Here's how the part is built. I have some questions about the finished solid (model axes, mm). A direction names the side the tool comes from. Coordinates: 2 decimals unless noted, no trailing zeros. Order: outer loops, then holes, each group sorted by start corner. A loop starts at its lowest first (then second) coordinate and runs counter-clockwise, first axis right, second up.
```python
from build123d import *

# Parameters (mm, degrees)
F1_DEPTH = 19.05
F2_W     = 44.4994677836
F2_H     = 19.1223323345
F3_DEPTH = 63.5
F5_DEPTH = 19.05
F6_DEPTH = 19.05


with BuildPart() as f1:
    # F0 (on Right) → F1 (new body)
    with BuildSketch(Plane.YZ):
        Polygon((-30.6730988776, 12.7), (-30.6730988776, 0), (32.876368906, 0), (32.876368906, 44.45), (13.826368906, 44.45), align=None)
    extrude(amount=F1_DEPTH)

    # F2 (on face) → F3 (join)
    with BuildSketch(Plane.YZ.offset(19.05)):
        with Locations((10.6266350142, 9.5611661673)):
            Rectangle(F2_W, F2_H)
    extrude(amount=F3_DEPTH)

    # F4 (on face) → F5 (join)
    with BuildSketch(Plane.YZ.offset(82.55)):
        Polygon((-11.6230988776, 19.1223323345), (32.876368906, 19.1223323345), (32.876368906, 44.45), (13.826368906, 44.45), (-30.623631094, 12.7), (-30.623631094, 0), (-11.6230988776, 0), align=None)
    extrude(amount=F5_DEPTH)

    # F6 (add, through all): a face of the model
    f6_faces = [f1.faces().sort_by_distance(p)[0] for p in [
        (82.55, 10.6266350142, 9.5611661673),
    ]]
    extrude(f6_faces, amount=F6_DEPTH)


solid = f1.part
```
Q1. If we section it at D-D on z = 10.5: Write out the boundary of the cut face in (x, y).
Q2. We'd pull the mould along X, two halves only. Please class faces 1 (the flat face through (101.6, 8, 18)), 2 (the flat face through (50, 10, 19.122)), 3 (the flat face through (50, 8, 0)): pulls with the +X half, pulls with the -X half, needs draft (parallel to the pull), parting line crosses it, or undercut.
Q3. For faces 4 (the flat face through (92, 23, 44.45)), 5 (the flat face through (50, -11.623, 9)), 6 (the flat face through (19.05, 1, 23)), which set-ups out of +Z, -Z, +X, -X, +Y, -Y let a thin tool reach every point of the face, with its end or its side?
Q4. If we section it at C-C on x = 94: Write out the boundary of the cut face in (y, z), then the cut area to 3 significant figures.
Q5. I need wall thicknesses on L1, parallel to X at y = 5, z = 27; L2, parallel to Y at x = 64.5, z = 3; L3, parallel to Z at x = 73, y = 11.5. Which ranges of each line are inside material? Lowest first, please.
Q6. If we section it at A-A on z = 40.5: Write out the boundary of the cut face in (x, y).
Q7. If we section it at B-B on y = 15.5: Write out the boundary of the cut face in (x, z).
Q8. Will these pins go through, and if not, where does the flat tip stop? pin 1 (15.5 mm diameter, centred on x = 52.5, z = 10, fed in from -Y); pin 2 (12 mm diameter, centred on x = 84, z = 14.5, fed in from -Y).
Reply:
1. outline: (0, -30.67) - (19.05, -30.67) - (19.05, -11.62) - (82.55, -11.62) - (82.55, -30.62) - (101.6, -30.62) - (101.6, 32.88) - (0, 32.88) - close
2. face 1: pulls with the +X half
2. face 2: undercut
2. face 3: needs draft
3. face 4: +Z, +X, -X, +Y, -Y
3. face 5: +Z, -Z, -Y
3. face 6: +Z, -Y
4. outline: (-30.62, 0) - (32.88, 0) - (32.88, 44.45) - (13.83, 44.45) - (-30.62, 12.7) - close
4. area: 2,120 mm2
5. L1: x = 0 to 19.05, 82.55 to 101.6
5. L2: y = -11.62 to 32.88
5. L3: z = 0 to 19.12
6. outline: (0, 8.29) - (19.05, 8.29) - (19.05, 32.88) - (0, 32.88) - close; (82.55, 8.3) - (101.6, 8.3) - (101.6, 32.88) - (82.55, 32.88) - close
7. outline: (0, 0) - (101.6, 0) - (101.6, 44.45) - (82.55, 44.45) - (82.55, 19.12) - (19.05, 19.12) - (19.05, 44.45) - (0, 44.45) - close
8. pin 1: stops at y = -11.62
8. pin 2: stops at y = -30.62
